```python
from build123d import *

# Parameters (mm, degrees)
SKETCH1_W           = 50
SKETCH1_H           = 37.5
BOSS_EXTRUDE1_DEPTH = 3
SKETCH2_W           = 15.1
SKETCH2_H           = 3.05
CUT_EXTRUDE1_DEPTH  = 32.393669744
CUT_EXTRUDE2_DEPTH  = 32.393669744
SKETCH4_W           = 3.1
SKETCH4_H           = 11.25
CUT_EXTRUDE3_DEPTH  = 32.393669744
SKETCH5_R           = 1.85
CUT_EXTRUDE4_DEPTH  = 32.393669744


with BuildPart() as part:
    # Sketch1 → Boss-Extrude1 (new body)
    with BuildSketch(Plane(origin=(0, 0, 0), x_dir=(1, 0, 0), z_dir=(0, 1, 0))):
        Rectangle(SKETCH1_W, SKETCH1_H)
    extrude(amount=BOSS_EXTRUDE1_DEPTH)

    # Sketch2 → Cut-Extrude1 (cut, through all)
    with BuildSketch(Plane(origin=(0, 3, 0), x_dir=(1, 0, 0), z_dir=(0, 1, 0))):
        with Locations((-0.05, -13.225)):
            Rectangle(SKETCH2_W, SKETCH2_H)
    extrude(amount=-CUT_EXTRUDE1_DEPTH, mode=Mode.SUBTRACT)

    # Sketch3 → Cut-Extrude2 (cut, through all)
    with BuildSketch(Plane(origin=(0, 3, 0), x_dir=(1, 0, 0), z_dir=(0, 1, 0))):
        Polygon((25, 7.55), (21.95, 7.55), (21.95, 1.85), (17.95, 1.85), (17.95, 4.1), (15.05, 4.1), (15.05, 1.85), (12.15, 1.85), (12.15, 0), (25, 0), align=None)
    cut_extrude2 = extrude(amount=-CUT_EXTRUDE2_DEPTH, mode=Mode.SUBTRACT)

    # Mirror1: Cut-Extrude2 across plane
    add(cut_extrude2.mirror(Plane.XY), mode=Mode.SUBTRACT)

    # Sketch4 → Cut-Extrude3 (cut, through all)
    with BuildSketch(Plane.XZ):
        with Locations((-23.45, -13.125)):
            Rectangle(SKETCH4_W, SKETCH4_H)
        with Locations((-23.45, 13.125)):
            Rectangle(SKETCH4_W, SKETCH4_H)
    extrude(amount=-CUT_EXTRUDE3_DEPTH, mode=Mode.SUBTRACT)

    # Sketch5 → Cut-Extrude4 (cut, through all)
    with BuildSketch(Plane.XZ):
        with Locations((-23.5, 0)):
            Circle(SKETCH5_R)
    extrude(amount=-CUT_EXTRUDE4_DEPTH, mode=Mode.SUBTRACT)


solid = part.part
```
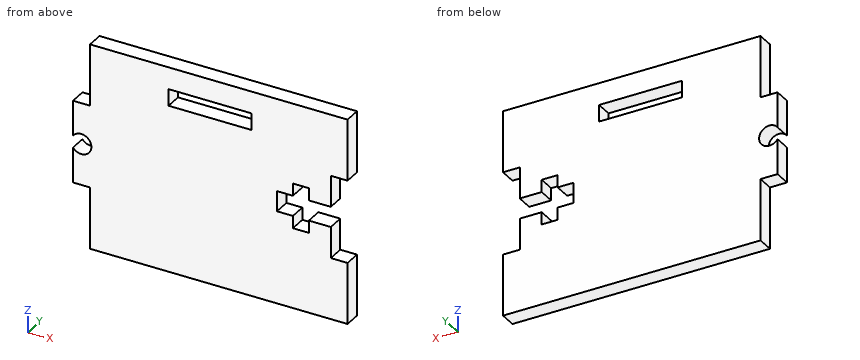
The model under review builds one solid part; all positions refer to its coordinate system, in mm. Round coordinates to 2 decimals unless told otherwise and drop trailing zeros. Order: outer loops, then holes, each group sorted by start corner. A loop starts at its lowest first (then second) coordinate and runs counter-clockwise, first axis right, second up. Notation, with made-up numbers: (9.5, -39.75) - (41.5, -39.75) arc R25 ccw to (41.5, -5.75) - close; hole circle Ø6 at (83.5, 17.5). An arc over 180 degrees is marked (long way). Answer in a Markdown table with one row per item.
(1) Take a section at A-A on x = 22.5. Write out the cut boundary in (y, z).
Result set:
| item | result |
|---|---|
| outline | (0, -18.75) - (3, -18.75) - (3, -7.55) - (0, -7.55) - close; (0, 7.55) - (3, 7.55) - (3, 18.75) - (0, 18.75) - close |
(2) For line 1 (Z direction, x = 3, y = 1.2); line 2 (Z direction, x = 21, y = 2.6); line 3 (X direction, y = 1.1, z = 12.5), list the stretches that pass through material, from the lowest coordinate up. Write a range as from..to.
Result set:
| item | result |
|---|---|
| line 1 | z = -18.75..11.7, 14.75..18.75 |
| line 2 | z = -18.75..-1.85, 1.85..18.75 |
| line 3 | x = -21.9..-7.6, 7.5..25 |
(3) Take a section at D-D on z = 0. Write out the cut boundary in (x, y).
Result set:
| item | result |
|---|---|
| outline | (-21.65, 0) - (12.15, 0) - (12.15, 3) - (-21.65, 3) - close |
(4) Take a section at C-C on z = 13.5. Write out the cut boundary in (x, y), plus the area to 3 significant figures.
Result set:
| item | result |
|---|---|
| outline | (-21.9, 0) - (-7.6, 0) - (-7.6, 3) - (-21.9, 3) - close; (7.5, 0) - (25, 0) - (25, 3) - (7.5, 3) - close |
| area | 95.4 mm2 |
(5) Clearance check with flat-ended pins moving along their axes: P1, Ø1.5, axis at x = -23, y = 2, coming from the +Z side; P2, Ø1.5, axis at y = 0.5, z = 12, coming from the -X side; P3, Ø2, axis at x = -23.5, z = 0, coming from the -Y side. State where each tip first meets the part, or that it passes through.
Result set:
| item | result |
|---|---|
| P1 | stops at z = 7.5 |
| P2 | stops at x = -21.9 |
| P3 | passes through |
